Could you check a few things on this model? Use its own coordinates, in mm. A direction names the side the tool comes from. Coordinates: 2 decimals unless noted, no trailing zeros. Loops run counter-clockwise (first coordinate to the right, second up) from the corner with the lowest first, then second, coordinate; pieces in that order, holes last.
1) Imagine slicing it at D-D on x = -20. Please give me the cut outline in (y, z).
2) If I drill on line 1 along Y through (x, z) = (0, 5.75); line 2 along X through (y, z) = (-49, 1); line 3 along X through (y, z) = (39.5, 5.25), over which ranges is the centre line in solid material (lowest first)?
3) Imagine slicing it at B-B on x = 0. Please give me the cut outline in (y, z).
4) For faces 1 (the face through (-26.726, -56.291, 5.07)), 2 (the face through (63, -5, 5)), 3 (the face through (-63, 5, 5)), which set-ups out of +Z, -Z, +X, -X, +Y, -Y let a thin tool reach every point of the face, with its end or its side?
5) Will these pins go through, and if not, where does the flat tip stop? P1, Ø6, axis at y = -3, z = 7.5, coming from the -X side; P2, Ø3, axis at y = 27, z = 5, coming from the -X side; P3, Ø3, axis at x = 70.5, z = 3.5, coming from the -Y side.
6) Imagine slicing it at A-A on y = 0. Please give me the cut outline in (x, z), plus the area to 3 significant figures.
7) Imagine slicing it at C-C on y = 60.5. Please give me the cut outline in (x, z), plus the area to 3 significant figures.
```python
from build123d import *

# Parameters (mm, degrees)
CROQUIS1_R              = 85
SALIENTE_EXTRUIR3_DEPTH = 10
CROQUIS3_R              = 10
CORTAR_EXTRUIR1_DEPTH   = 10
CORTAR_EXTRUIR2_DEPTH   = 10
MATRIZC1_COUNT          = 6
CROQUIS5_R              = 35
CORTAR_EXTRUIR3_DEPTH   = 10
MATRIZC2_COUNT          = 6


with BuildPart() as part:
    # Croquis1 → Saliente-Extruir3 (new body)
    with BuildSketch(Plane.XY):
        Circle(CROQUIS1_R)
    extrude(amount=SALIENTE_EXTRUIR3_DEPTH)

    # Croquis3 → Cortar-Extruir1 (cut)
    with BuildSketch(Plane.XY.offset(10)):
        Circle(CROQUIS3_R)
    extrude(amount=-CORTAR_EXTRUIR1_DEPTH, mode=Mode.SUBTRACT)

    # Croquis4 → Cortar-Extruir2 (cut)
    with BuildSketch(Plane.XY.offset(10)):
        with BuildLine():
            Line((40, 5), (99.874921777, 5))
            ThreePointArc((99.874921777, 5), (100, 0), (99.874921777, -5))
            Line((99.874921777, -5), (40, -5))
            ThreePointArc((40, -5), (35, 0), (40, 5))
        make_face()
    cortar_extruir2 = extrude(amount=-CORTAR_EXTRUIR2_DEPTH, mode=Mode.SUBTRACT)

    # MatrizC1: Cortar-Extruir2 ×6 about axis
    matrizc1_axis = Axis((0, 0, 0), (0, 0, 1))
    for i in range(1, MATRIZC1_COUNT):
        add(cortar_extruir2.rotate(matrizc1_axis, i * 360 / MATRIZC1_COUNT), mode=Mode.SUBTRACT)

    # Croquis5 → Cortar-Extruir3 (cut)
    with BuildSketch(Plane.XY.offset(10)):
        with Locations((86.602540378, 50)):
            Circle(CROQUIS5_R)
    cortar_extruir3 = extrude(amount=-CORTAR_EXTRUIR3_DEPTH, mode=Mode.SUBTRACT)

    # MatrizC2: Cortar-Extruir3 ×6 about axis
    matrizc2_axis = Axis((0, 0, 0), (0, 0, 1))
    for i in range(1, MATRIZC2_COUNT):
        add(cortar_extruir3.rotate(matrizc2_axis, i * 360 / MATRIZC2_COUNT), mode=Mode.SUBTRACT)


solid = part.part
```
Filled in:
1. outline: (-71.28, 0) - (-44.64, 0) - (-44.64, 10) - (-71.28, 10) - close; (-29.64, 0) - (29.64, 0) - (29.64, 10) - (-29.64, 10) - close; (44.64, 0) - (71.28, 0) - (71.28, 10) - (44.64, 10) - close
2. line 1: y = -65 to -10, 10 to 65
2. line 2: x = -51.62 to -34.06, -22.52 to 22.52, 34.06 to 51.62
2. line 3: x = -53.21 to -28.58, -17.03 to 17.03, 28.58 to 53.21
3. outline: (-65, 0) - (-10, 0) - (-10, 10) - (-65, 10) - close; (10, 0) - (65, 0) - (65, 10) - (10, 10) - close
4. face 1: +Z, -Z
4. face 2: +Z, -Z, +X
4. face 3: +Z, -Z, -X
5. P1: stops at x = -84.85
5. P2: stops at x = -61.61
5. P3: stops at y = -19.75
6. outline: (-35, 0) - (-10, 0) - (-10, 10) - (-35, 10) - close; (10, 0) - (35, 0) - (35, 10) - (10, 10) - close
6. area: 500 mm2
7. outline: (-53.21, 0) - (-40.7, 0) - (-40.7, 10) - (-53.21, 10) - close; (-29.16, 0) - (29.16, 0) - (29.16, 10) - (-29.16, 10) - close; (40.7, 0) - (53.21, 0) - (53.21, 10) - (40.7, 10) - close
7. area: 833 mm2
